The listing builds one solid part. Answer for the finished solid, in the listing's coordinates (mm). Face numbers are marked on the shaded views. Round coordinates to 2 decimals unless told otherwise and drop trailing zeros. Write each loop counter-clockwise with the first axis right and the second up, starting at its lowest first coordinate (ties: lowest second). Pieces come first, ordered by that corner, then holes. Notation, with made-up numbers: (86, 25.5) - (136, 25.5) arc R19 cw to (136, 56.5) - close; hole circle Ø9 at (-21.75, -30). An arc over 180 degrees is marked (long way). Return JSON: item names as keys, results as strings. Group by question number.
(1) Section A-A, the plane x = 0 is taken. Write down the section's boundary in (y, z) (1 decimal).
(2) Determine the mould class of the marked faces 1, 2 and 3 for opening direction Y: +Y half, -Y half, draft (parallel to the pull), parting line (faces both ways), or undercut.
(3) Each of these flat-tipped pins is pushed along its axis until it touches: pin 1 (1 mm diameter, centred on x = 0, z = 17.5, fed in from -Y); pin 2 (1 mm diameter, centred on x = -1, z = 12, fed in from +Y). Where does it stop, or does it pass through?
(4) Find the intervals of material crossed by line 1 along Y through (x, z) = (0, 4); line 2 along Z through (x, y) = (0.75, 3.25) (3 decimals); line 3 along Y through (x, z) = (2, 3.5), in increasing order. Write a range as [from, to].
(5) Section C-C, the plane z = 14.5 is taken. Write down the section's boundary in (x, y) (1 decimal), then the cut area to 3 significant figures.
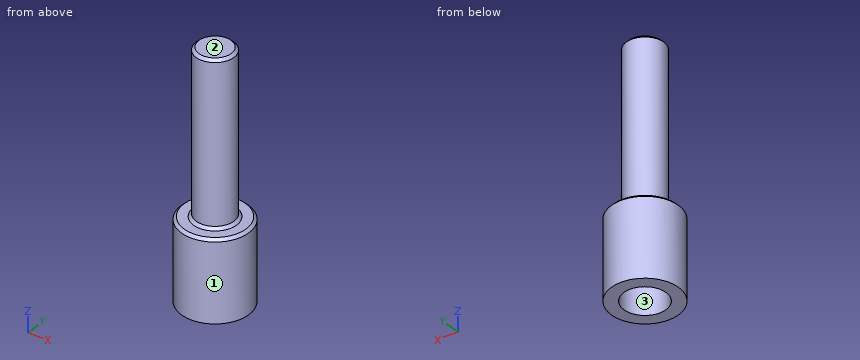
```python
from build123d import *

# Parameters (mm, degrees)
SKETCH1_R           = 3.96875
BOSS_EXTRUDE1_DEPTH = 28.575
CUT_EXTRUDE1_START  = -19.05
SKETCH2_R           = 3.96875
SKETCH2_R_2         = 2.2225
CUT_EXTRUDE1_DEPTH  = 19.05
SKETCH3_R           = 2.4892
CUT_EXTRUDE2_DEPTH  = 7.62
CHAMFER1_SIZE       = 0.3175


with BuildPart() as part:
    # Sketch1 → Boss-Extrude1 (new body)
    with BuildSketch(Plane.XY):
        Circle(SKETCH1_R)
    extrude(amount=BOSS_EXTRUDE1_DEPTH)

    # Sketch2 → Cut-Extrude1 (cut)
    with BuildSketch(Plane.XY.offset(28.575).offset(CUT_EXTRUDE1_START)):
        Circle(SKETCH2_R)
        Circle(SKETCH2_R_2, mode=Mode.SUBTRACT)
    extrude(amount=CUT_EXTRUDE1_DEPTH, mode=Mode.SUBTRACT)

    # Sketch3 → Cut-Extrude2 (cut)
    with BuildSketch(Plane(origin=(0, 0, 0), x_dir=(-1, 0, 0), z_dir=(0, 0, -1))):
        Circle(SKETCH3_R)
    extrude(amount=-CUT_EXTRUDE2_DEPTH, mode=Mode.SUBTRACT)

    # Chamfer1
    chamfer1_edges = [part.edges().sort_by_distance(p)[0] for p in [
        (-2.2225, 0, 28.575),
        (-3.96875, 0, 9.525),
        (-2.2225, 0, 9.525),
    ]]
    chamfer(chamfer1_edges, length=CHAMFER1_SIZE)


solid = part.part
```
Working result:
{
 "1": {"outline": "(-4, 0) - (-2.5, 0) - (-2.5, 7.6) - (2.5, 7.6) - (2.5, 0) - (4, 0) - (4, 9.2) - (3.7, 9.5) - (2.5, 9.5) - (2.2, 9.8) - (2.2, 28.3) - (1.9, 28.6) - (-1.9, 28.6) - (-2.2, 28.3) - (-2.2, 9.8) - (-2.5, 9.5) - (-3.7, 9.5) - (-4, 9.2) - close"},
 "2": {"face 1": "parting line", "face 2": "draft", "face 3": "undercut"},
 "3": {"pin 1": "stops at y = -2.22", "pin 2": "stops at y = 2.17"},
 "4": {"line 1": "y = [-3.97, -2.49], [2.49, 3.97]", "line 2": "z = [0, 9.525]", "line 3": "y = [-3.43, -1.48], [1.48, 3.43]"},
 "5": {"outline": "circle Ø4.4 at (0, 0)", "area": "15.5 mm^2"}
}
